```python
from build123d import *

# Parameters (mm, degrees)
SKETCH1_R           = 5
BOSS_EXTRUDE1_DEPTH = 200
CHAMFER1_SIZE       = 1
BOSS_EXTRUDE3_START = 70
SKETCH2_R           = 7
BOSS_EXTRUDE3_DEPTH = 10


with BuildPart() as part:
    # Sketch1 → Boss-Extrude1 (new body)
    with BuildSketch(Plane(origin=(0, 0, 0), x_dir=(0, 0, -1), z_dir=(1, 0, 0))):
        Circle(SKETCH1_R)
    extrude(amount=BOSS_EXTRUDE1_DEPTH)

    # Chamfer1
    chamfer1_edges = [part.edges().sort_by_distance(p)[0] for p in [
        (0, 0, 5),
        (200, 0, 5),
    ]]
    chamfer(chamfer1_edges, length=CHAMFER1_SIZE)

    # Sketch2 → Boss-Extrude3 (add)
    with BuildSketch(Plane(origin=(0, 0, 0), x_dir=(0, 0, -1), z_dir=(1, 0, 0)).offset(BOSS_EXTRUDE3_START)):
        Circle(SKETCH2_R)
    extrude(amount=BOSS_EXTRUDE3_DEPTH)


solid = part.part
```
The listing builds one solid part. Answer for the finished solid, in the listing's coordinates (mm). A direction names the side the tool comes from. Coordinates: 2 decimals unless noted, no trailing zeros. Loops run counter-clockwise (first coordinate to the right, second up) from the corner with the lowest first, then second, coordinate; pieces in that order, holes last. Notation, with made-up numbers: (55.25, 4) -> (104.25, 4) arc R21 cw to (104.25, 20) -> close; hole circle Ø2 at (0, -2). An arc over 180 degrees is marked (long way). Use one line per item in the form item = value. Start each with the question number.
Item 1: The part is cut by section C-C on x = 131. Determine the outline of the cut face in (y, z).
Item 2: A tool of negligible diameter and unlimited length cuts with its end or side. For faces 1 (the face through (35.02, -4.88, 1.08)), 2 (the face through (80, 5, 2)), 3 (the face through (200, 0, 0)), from which of +Z, -Z, +X, -X, +Y, -Y can it reach the whole face along a straight path? Write none if from no direction.
Item 3: Flat-ended cylindrical pins translate along their axes: pin 1 Ø8 at (x, y) = (52, 0) entering from +Z; pin 2 Ø1 at (x, y) = (41, 3.5) entering from +Z; pin 3 Ø6 at (x, z) = (157, 0) entering from +Y. Find the tip coordinate at first contact, or state that the pin passes through.
Item 4: Consider L1, parallel to X at y = -5.25, z = -3.5; L2, parallel to X at y = 1.5, z = -3.75; L3, parallel to Z at x = 48.5, y = 0. Determine where each line is inside the solid, lowest interval first. Write a range as [from, to].
Item 5: The part is cut by section A-A on z = 0. Determine the outline of the cut face in (x, y).
Answer key:
q1.outline = circle Ø10 at (0, 0)
q2.face_1 = -X
q2.face_2 = +X
q2.face_3 = +Z, -Z, +X, +Y, -Y
q3.pin_1 = 5
q3.pin_2 = 4
q3.pin_3 = 5
q4.L1 = [70, 80]
q4.L2 = [0.04, 199.96]
q4.L3 = [-5, 5]
q5.outline = (0, -4) -> (1, -5) -> (70, -5) -> (70, -7) -> (80, -7) -> (80, -5) -> (199, -5) -> (200, -4) -> (200, 4) -> (199, 5) -> (80, 5) -> (80, 7) -> (70, 7) -> (70, 5) -> (1, 5) -> (0, 4) -> close
